from build123d import *

# Parameters (mm, degrees)
F0_W     = 197.273388
F0_H     = 100.243152
F1_DEPTH = 38.1
F3_DEPTH = 100.244151
F5_DEPTH = 6.35
F7_DEPTH = 6.35


with BuildPart() as f1:
    # F0 (on Top) → F1 (new body)
    with BuildSketch(Plane.XY):
        Rectangle(F0_W, F0_H)
    extrude(amount=F1_DEPTH)

    # F2 (on face) → F3 (cut, through all)
    with BuildSketch(Plane.XZ.offset(50.121576)):
        Polygon((98.636694, 38.1), (-98.636694, 38.1), (0, 5.87702), (98.636694, 5.87702), align=None)
    extrude(amount=-F3_DEPTH, mode=Mode.SUBTRACT)

    # F4 (on face) → F5 (join)
    with BuildSketch(Plane.XZ.offset(50.121576)):
        Polygon((-98.636694, 49.251463), (-98.636694, 0), (98.636694, 0), (98.636694, 11.338987), (0, 11.338987), align=None)
    extrude(amount=F5_DEPTH)

    # F6 (on face) → F7 (join)
    with BuildSketch(Plane(origin=(0, 50.121576, 0), x_dir=(-1, 0, 0), z_dir=(0, 1, 0))):
        Polygon((-98.636694, 0), (98.636694, 0), (98.636694, 49.251463), (0, 11.338987), (-98.636694, 11.338987), align=None)
    extrude(amount=F7_DEPTH)


solid = f1.part
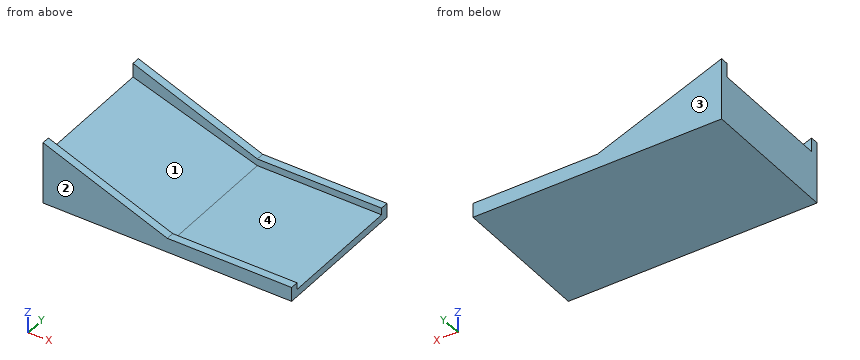
Part model, mm, in its own coordinate system. Face numbers are marked on the shaded views. Coordinates: 2 decimals unless noted, no trailing zeros. Write each loop counter-clockwise with the first axis right and the second up, starting at its lowest first coordinate (ties: lowest second). Pieces come first, ordered by that corner, then holes. Notation, with made-up numbers: M 7.25,77.25 L 44.25,77.25 A7 cw 44.25,84.25 Z; hole C 12,9.25 d5. An arc over 180 degrees is marked long. Return JSON: item names as keys, results as strings.
1. Saw through at C-C, the plane x = 27. Write the cut outline in (y, z).
Determined:
{"outline": "M -56.47,0 L 56.47,0 L 56.47,11.34 L 50.12,11.34 L 50.12,5.88 L -50.12,5.88 L -50.12,11.34 L -56.47,11.34 Z"}
2. Saw through at B-B, the plane y = 26. Write the cut outline in (x, z).
Determined:
{"outline": "M -98.64,0 L 98.64,0 L 98.64,5.88 L 0,5.88 L -98.64,38.1 Z"}
3. Saw through at D-D, the plane z = 32.5. Write the cut outline in (x, y), then the cut area to 3 significant figures.
Determined:
{"outline": "M -98.64,-56.47 L -55.05,-56.47 L -55.05,-50.12 L -81.49,-50.12 L -81.49,50.12 L -55.05,50.12 L -55.05,56.47 L -98.64,56.47 Z", "area": "2,270 mm²"}
4. Probe L1, parallel to Z at x = 17.5, y = 3.5; L2, parallel to Z at x = -60.5, y = -49.5. List the from-to ranges inside material, lowest first.
Determined:
{"L1": "0 to 5.88", "L2": "0 to 25.64"}
5. Saw through at A-A, the plane z = 43. Write the cut outline in (x, y).
Determined:
{"outline": "M -98.64,-56.47 L -82.37,-56.47 L -82.37,-50.12 L -98.64,-50.12 Z; M -98.64,50.12 L -82.37,50.12 L -82.37,56.47 L -98.64,56.47 Z"}
6. Pull direction Y, two halves, no side cores. Call the marked faces 1, 2, 3 and 4: pulls with the +Y half, pulls with the -Y half, needs draft (parallel to the pull), parting line crosses it, or undercut.
Determined:
{"face 1": "undercut", "face 2": "pulls with the -Y half", "face 3": "pulls with the +Y half", "face 4": "undercut"}
7. Flat gauge pins, fed straight in: pin 1 Ø3 at (x, y) = (65, -54.5) entering from +Z; pin 2 Ø1.5 at (x, y) = (-35.5, -8) entering from +Z. Where does each tip first touch, or does it go through?
Determined:
{"pin 1": "z = 11.34", "pin 2": "z = 17.72"}
